Work out the finished part from the listing and answer in its coordinate system (mm). Round coordinates to 2 decimals unless told otherwise and drop trailing zeros. Loops run counter-clockwise (first coordinate to the right, second up) from the corner with the lowest first, then second, coordinate; pieces in that order, holes last. Notation, with made-up numbers: (22, 64.25) - (49, 64.25) arc R17 ccw to (49, 83.25) - close; hole circle Ø6 at (41.5, 12.25). An arc over 180 degrees is marked (long way). Return JSON: item names as keys, results as strings.
from build123d import *
from OCP.BRepFilletAPI import BRepFilletAPI_MakeChamfer

# Parameters (mm, degrees)
SKETCH2_R          = 2.5
CUT_EXTRUDE1_DEPTH = 5
CUT_EXTRUDE2_DEPTH = 5
CHAMFER2_SIZE      = 0.5
CHAMFER2_SIZE_2    = 1


with BuildPart() as part:
    # Sketch1 → Revolve1 (revolve)
    with BuildSketch(Plane(origin=(0, 0, 0), x_dir=(0, 0, -1), z_dir=(1, 0, 0))):
        with BuildLine():
            Line((0, 0), (0, -8.5))
            ThreePointArc((0, -8.5), (-6.01040764, -6.01040764), (-8.5, 0))
            Line((-8.5, 0), (0, 0))
        make_face()
    revolve(axis=Axis((0, 0, 0), (0, 0, 1)))

    # Sketch2 → Cut-Extrude1 (cut)
    with BuildSketch(Plane(origin=(0, 0, 0), x_dir=(-1, 0, 0), z_dir=(0, 0, -1))):
        with Locations(Location((0, 0, 0), (0, 0, 90))):
            Circle(SKETCH2_R)
    extrude(amount=-CUT_EXTRUDE1_DEPTH, mode=Mode.SUBTRACT)

    # Sketch3 → Cut-Extrude2 (cut)
    with BuildSketch(Plane(origin=(0, 0, 0), x_dir=(-1, 0, 0), z_dir=(0, 0, -1))):
        with BuildLine():
            ThreePointArc((-0.75, 2.90473751), (-1.5, 2.598076211), (-2.140576475, 2.101887808))
            Line((-2.140576475, 2.101887808), (-1.690338955, 1.841943055))
            ThreePointArc((-1.690338955, 1.841943055), (-1.25, 2.165063509), (-0.75, 2.384848004))
            Line((-0.75, 2.384848004), (-0.75, 2.90473751))
        make_face()
        with BuildLine():
            Line((1.690338955, 1.841943055), (2.140576475, 2.101887808))
            ThreePointArc((2.140576475, 2.101887808), (1.5, 2.598076211), (0.75, 2.90473751))
            Line((0.75, 2.90473751), (0.75, 2.384848004))
            ThreePointArc((0.75, 2.384848004), (1.25, 2.165063509), (1.690338955, 1.841943055))
        make_face()
        with BuildLine():
            Line((2.440338955, -0.542904949), (2.890576475, -0.802849702))
            ThreePointArc((2.890576475, -0.802849702), (2.972518244, -0.405136135), (3, 0))
            ThreePointArc((3, 0), (2.972518244, 0.405136135), (2.890576475, 0.802849702))
            Line((2.890576475, 0.802849702), (2.440338955, 0.542904949))
            ThreePointArc((2.440338955, 0.542904949), (2.485039978, 0.273086627), (2.5, 0))
            ThreePointArc((2.5, 0), (2.485039978, -0.273086627), (2.440338955, -0.542904949))
        make_face()
        with BuildLine():
            Line((0.75, -2.384848004), (0.75, -2.90473751))
            ThreePointArc((0.75, -2.90473751), (1.5, -2.598076211), (2.140576475, -2.101887808))
            Line((2.140576475, -2.101887808), (1.690338955, -1.841943055))
            ThreePointArc((1.690338955, -1.841943055), (1.25, -2.165063509), (0.75, -2.384848004))
        make_face()
        with BuildLine():
            ThreePointArc((-2.140576475, -2.101887808), (-1.5, -2.598076211), (-0.75, -2.90473751))
            Line((-0.75, -2.90473751), (-0.75, -2.384848004))
            ThreePointArc((-0.75, -2.384848004), (-1.25, -2.165063509), (-1.690338955, -1.841943055))
            Line((-1.690338955, -1.841943055), (-2.140576475, -2.101887808))
        make_face()
        with BuildLine():
            ThreePointArc((-2.890576475, 0.802849702), (-3, 0), (-2.890576475, -0.802849702))
            Line((-2.890576475, -0.802849702), (-2.440338955, -0.542904949))
            ThreePointArc((-2.440338955, -0.542904949), (-2.5, 0), (-2.440338955, 0.542904949))
            Line((-2.440338955, 0.542904949), (-2.890576475, 0.802849702))
        make_face()
    extrude(amount=-CUT_EXTRUDE2_DEPTH, mode=Mode.SUBTRACT)

    # Chamfer2
    chamfer2_edges_1 = [part.edges().sort_by_distance(p)[0] for p in [
        (-2.165063509, 1.25, 0),
    ]]
    chamfer2_side_1 = [part.faces().sort_by_distance(p)[0] for p in [
        (-2.173723763, 1.255, 0),
    ]]
    chamfer2_edges_2 = [part.edges().sort_by_distance(p)[0] for p in [
        (2.165063509, -1.25, 0),
    ]]
    chamfer2_side_2 = [part.faces().sort_by_distance(p)[0] for p in [
        (2.173723763, -1.255, 0),
    ]]
    chamfer2_edges_3 = [part.edges().sort_by_distance(p)[0] for p in [
        (0, 2.5, 0),
    ]]
    chamfer2_side_3 = [part.faces().sort_by_distance(p)[0] for p in [
        (0, 2.51, 0),
    ]]
    chamfer2_edges_4 = [part.edges().sort_by_distance(p)[0] for p in [
        (0, -2.5, 0),
    ]]
    chamfer2_side_4 = [part.faces().sort_by_distance(p)[0] for p in [
        (0, -2.51, 0),
    ]]
    chamfer2_edges_5 = [part.edges().sort_by_distance(p)[0] for p in [
        (2.165063509, 1.25, 0),
    ]]
    chamfer2_side_5 = [part.faces().sort_by_distance(p)[0] for p in [
        (2.173723763, 1.255, 0),
    ]]
    chamfer2_edges_6 = [part.edges().sort_by_distance(p)[0] for p in [
        (-2.165063509, -1.25, 0),
    ]]
    chamfer2_side_6 = [part.faces().sort_by_distance(p)[0] for p in [
        (-2.173723763, -1.255, 0),
    ]]
    chamfer2 = BRepFilletAPI_MakeChamfer(part.part.solid().wrapped)
    for e in chamfer2_edges_1:
        chamfer2.Add(CHAMFER2_SIZE - 0.0001, CHAMFER2_SIZE_2 - 0.0001, e.wrapped, chamfer2_side_1[0].wrapped)
    for e in chamfer2_edges_2:
        chamfer2.Add(CHAMFER2_SIZE - 0.0001, CHAMFER2_SIZE_2 - 0.0001, e.wrapped, chamfer2_side_2[0].wrapped)
    for e in chamfer2_edges_3:
        chamfer2.Add(CHAMFER2_SIZE - 0.0001, CHAMFER2_SIZE_2 - 0.0001, e.wrapped, chamfer2_side_3[0].wrapped)
    for e in chamfer2_edges_4:
        chamfer2.Add(CHAMFER2_SIZE - 0.0001, CHAMFER2_SIZE_2 - 0.0001, e.wrapped, chamfer2_side_4[0].wrapped)
    for e in chamfer2_edges_5:
        chamfer2.Add(CHAMFER2_SIZE - 0.0001, CHAMFER2_SIZE_2 - 0.0001, e.wrapped, chamfer2_side_5[0].wrapped)
    for e in chamfer2_edges_6:
        chamfer2.Add(CHAMFER2_SIZE - 0.0001, CHAMFER2_SIZE_2 - 0.0001, e.wrapped, chamfer2_side_6[0].wrapped)
    add(Compound.cast(chamfer2.Shape()), mode=Mode.REPLACE)  # a hair under: the kernel refuses the full size


solid = part.part
1) Find the intervals of material crossed by L1, parallel to X at y = 1.5, z = 1.25; L2, parallel to Y at x = 2.25, z = 2; L3, parallel to X at y = -1.75, z = 1.25, in increasing order.
Verdict:
{"L1": "x = -8.27 to -2, 2 to 8.27", "L2": "y = -7.95 to -1.09, 1.09 to 7.95", "L3": "x = -8.22 to -1.79, 1.79 to 8.22"}
2) Section B-B (z = 7.5) is taken. Give the vertices of the cut face in (x, y), and give its area (3 significant figures).
Verdict:
{"outline": "circle Ø8 at (0, 0)", "area": "50.3 mm2"}
3) Section A-A (z = 2.5) is taken. Give the vertices of the cut face in (x, y).
Verdict:
{"outline": "circle Ø16.25 at (0, 0); hole (-2.89, -0.8) - (-2.44, -0.54) arc R2.5 ccw to (-1.69, -1.84) - (-2.14, -2.1) arc R3 ccw to (-0.75, -2.9) - (-0.75, -2.38) arc R2.5 ccw to (0.75, -2.38) - (0.75, -2.9) arc R3 ccw to (2.14, -2.1) - (1.69, -1.84) arc R2.5 ccw to (2.44, -0.54) - (2.89, -0.8) arc R3 ccw to (2.89, 0.8) - (2.44, 0.54) arc R2.5 ccw to (1.69, 1.84) - (2.14, 2.1) arc R3 ccw to (0.75, 2.9) - (0.75, 2.38) arc R2.5 ccw to (-0.75, 2.38) - (-0.75, 2.9) arc R3 ccw to (-2.14, 2.1) - (-1.69, 1.84) arc R2.5 ccw to (-2.44, 0.54) - (-2.89, 0.8) arc R3 ccw to start"}
4) Section D-D (x = 7.5) is taken. Give the vertices of the cut face in (y, z), and give its area (3 significant figures).
Verdict:
{"outline": "(-4, 0) - (4, 0) arc R4 ccw to start", "area": "25.1 mm2"}
5) Section C-C (y = -4) is taken. Give the vertices of the cut face in (x, z).
Verdict:
{"outline": "(-7.5, 0) - (7.5, 0) arc R7.5 ccw to start"}
6) Flat-ended cylindrical pins translate along their axes: pin 1 (4 mm diameter, centred on x = -3, z = 4, fed in from -Y); pin 2 (1 mm diameter, centred on x = 5.5, z = 3.5, fed in from +Y); pin 3 (3 mm diameter, centred on x = -2.5, z = 3, fed in from -Y). Find the tip coordinate at first contact, or state that the pin passes through.
Verdict:
{"pin 1": "stops at y = -7.95", "pin 2": "stops at y = 6", "pin 3": "stops at y = -8.15"}
7) Determine the mould class of faces 1 (the cylindrical face through (2.17, -1.24, 2.97)), 2 (the flat face through (0, 4, 0)) for opening direction Y: pulls with the +Y half, pulls with the -Y half, needs draft (parallel to the pull), parting line crosses it, or undercut.
Verdict:
{"face 1": "undercut", "face 2": "needs draft"}
